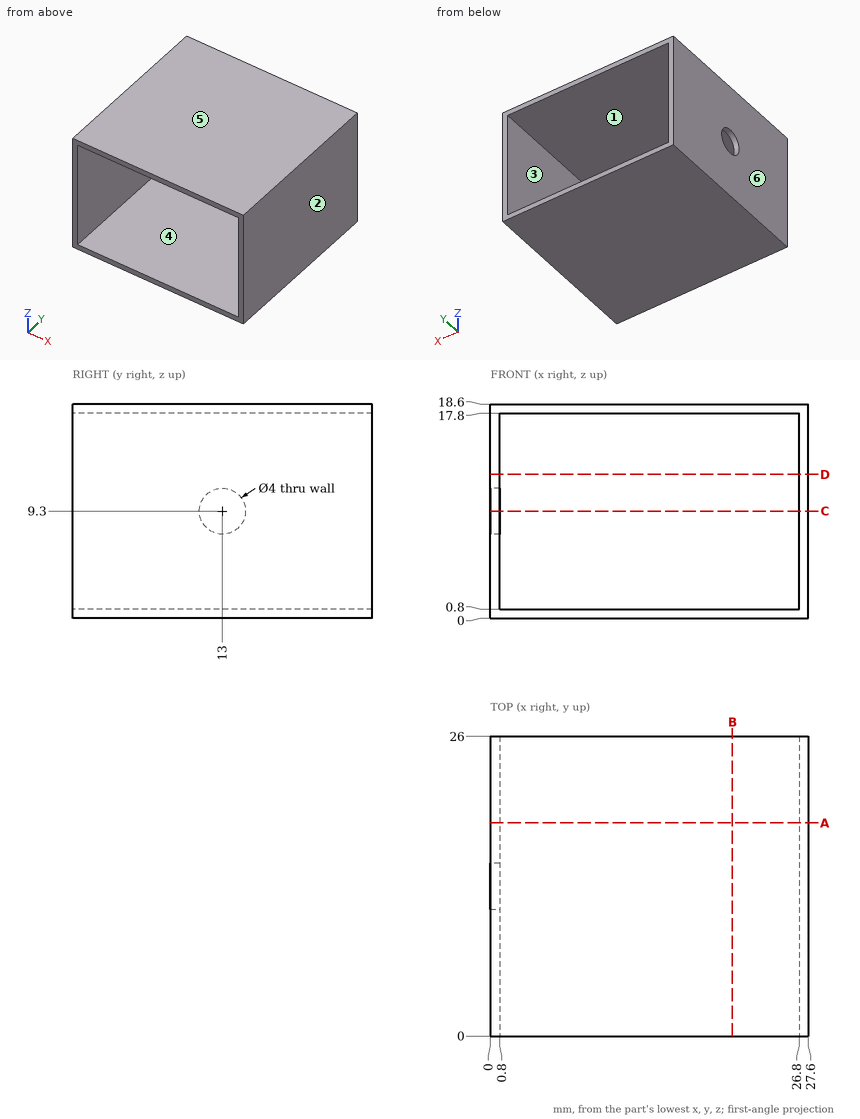
Could you check a few things on this drawing? It's one solid part, dimensions in mm from its lowest x, y, z. A direction names the side the tool comes from. Coordinates: 2 decimals unless noted, no trailing zeros. Order: outer loops, then holes, each group sorted by start corner. A loop starts at its lowest first (then second) coordinate and runs counter-clockwise, first axis right, second up. Notation, with made-up numbers: (13.5, 12) -> (66.5, 12) arc R12 ccw to (66.5, 33) -> close; hole circle Ø4 at (46, -38.5). An arc over 180 degrees is marked (long way). One line per item, written item: value. Start each with the question number.
1) Imagine slicing it at A-A on y = 18.5. List the corners of the cut face in (x, z) for me.
2) Imagine slicing it at C-C on z = 9.3. List the corners of the cut face in (x, y) for me, plus the area to 3 significant figures.
3) Imagine slicing it at B-B on x = 21. List the corners of the cut face in (y, z) for me.
4) We'd pull the mould along Z, two halves only. Please class the marked faces 3, 4, 5 and 6: +Z half, -Z half, draft (parallel to the pull), parting line (faces both ways), or undercut.
5) Which directions (+Z, -Z, +X, -X, +Y, -Y) give clear straight access to the entire face, cutting with the end or side of a thin tool? Please do the marked faces 1 and 2.
6) If I drill on L1, parallel to Z at x = 23.25, y = 2.25; L2, parallel to Z at x = 0.5, y = 13; L3, parallel to X at y = 10.75, z = 6, over which ranges is the centre line in solid material (lowest first)? Write a range as [from, to].
7) Imagine slicing it at D-D on z = 12.5. List the corners of the cut face in (x, y) for me, plus the area to 3 significant figures.
Answer list:
1. outline: (0, 0) -> (27.6, 0) -> (27.6, 18.6) -> (0, 18.6) -> close; hole (0.8, 0.8) -> (26.8, 0.8) -> (26.8, 17.8) -> (0.8, 17.8) -> close
2. outline: (0, 0) -> (0.8, 0) -> (0.8, 11) -> (0, 11) -> close; (0, 15) -> (0.8, 15) -> (0.8, 26) -> (0, 26) -> close; (26.8, 0) -> (27.6, 0) -> (27.6, 26) -> (26.8, 26) -> close
2. area: 38.4 mm2
3. outline: (0, 0) -> (26, 0) -> (26, 0.8) -> (0, 0.8) -> close; (0, 17.8) -> (26, 17.8) -> (26, 18.6) -> (0, 18.6) -> close
4. face 3: undercut
4. face 4: undercut
4. face 5: +Z half
4. face 6: draft
5. face 1: +Y, -Y
5. face 2: +Z, -Z, +X, +Y, -Y
6. L1: z = [0, 0.8], [17.8, 18.6]
6. L2: z = [0, 7.3], [11.3, 18.6]
6. L3: x = [0, 0.8], [26.8, 27.6]
7. outline: (0, 0) -> (0.8, 0) -> (0.8, 26) -> (0, 26) -> close; (26.8, 0) -> (27.6, 0) -> (27.6, 26) -> (26.8, 26) -> close
7. area: 41.6 mm2
